```python
from build123d import *

# Parameters (mm, degrees)
F0_W      = 173
F0_H      = 50
F1_DEPTH  = 1.5
F2_W      = 1.5
F2_H      = 4.5
F4_DEPTH  = 1.501
F3_W      = 1.5
F3_H      = 4.5
F5_DEPTH  = 1.501
F6_W      = 4
F6_H      = 2.7
F7_DEPTH  = 1.501
F8_R      = 1.35
F9_DEPTH  = 1.501
F10_R     = 3.75
F11_DEPTH = 1.501
F12_W     = 4
F12_H     = 1.2
F13_DEPTH = 1.501
F14_W     = 1.4
F14_H     = 4
F15_DEPTH = 1.501
F16_R     = 1
F17_R     = 0.5
F18_DEPTH = 1.501
F19_W     = 1.5543582849
F19_H     = 10.2004739456
F20_DEPTH = 1.501


# Not quite as in the source:
# - a pattern or mirror of a feature is missing from the dataset's text; its kind, count and spacing are read off the source's solid


with BuildPart() as f1:
    # F0 (on Top) → F1 (new body)
    with BuildSketch(Plane.XY):
        Rectangle(F0_W, F0_H)
    extrude(amount=F1_DEPTH)

    # F2 (on face) → F4 (cut, through all)
    with BuildSketch(Plane.XY.offset(1.5)):
        with Locations((-69.95, 2.75)):
            Rectangle(F2_W, F2_H)
    extrude(amount=-F4_DEPTH, mode=Mode.SUBTRACT)

    # F3 (on face) → F5 (cut, through all)
    with BuildSketch(Plane.XY.offset(1.5)):
        with Locations((-55.25, 2.75)):
            Rectangle(F3_W, F3_H)
    extrude(amount=-F5_DEPTH, mode=Mode.SUBTRACT)

    # F6 (on face) → F7 (cut, through all)
    with BuildSketch(Plane.XY.offset(1.5)):
        with Locations((-18.5, 20.65)):
            Rectangle(F6_W, F6_H)
    f7 = extrude(amount=-F7_DEPTH, mode=Mode.SUBTRACT)

    # F7_copies: F7 across plane
    add(f7.mirror(Plane(origin=(0, 0, 0), x_dir=(0, 0, -1), z_dir=(0, -1, 0))), mode=Mode.SUBTRACT)

    # F8 (on face) → F9 (cut, through all)
    with BuildSketch(Plane.XY.offset(1.5)):
        with Locations((56.55, 20.45)):
            Circle(F8_R)
    f9 = extrude(amount=-F9_DEPTH, mode=Mode.SUBTRACT)

    # F9_copies: F9 across plane
    add(f9.mirror(Plane(origin=(0, 0, 0), x_dir=(0, 0, -1), z_dir=(0, -1, 0))), mode=Mode.SUBTRACT)

    # F10 (on face) → F11 (cut, through all)
    with BuildSketch(Plane.XY.offset(1.5)):
        with Locations((76.35, 16.45)):
            Circle(F10_R)
        with Locations((76.35, -11.75)):
            Circle(F10_R)
    extrude(amount=-F11_DEPTH, mode=Mode.SUBTRACT)

    # F12 (on face) → F13 (cut, through all)
    with BuildSketch(Plane.XY.offset(1.5)):
        with Locations((84.5, 8.2552298188)):
            Rectangle(F12_W, F12_H)
        with Locations((84.5, -2.9447701812)):
            Rectangle(F12_W, F12_H)
    extrude(amount=-F13_DEPTH, mode=Mode.SUBTRACT)

    # F14 (on face) → F15 (cut, through all)
    with BuildSketch(Plane.XY.offset(1.5)):
        with Locations((75.6, 2.8)):
            Rectangle(F14_W, F14_H)
    extrude(amount=-F15_DEPTH, mode=Mode.SUBTRACT)

    # F16
    f16_edges = [f1.edges().sort_by_distance(p)[0] for p in [
        (-86.5, -25, 0.75),
        (-86.5, 25, 0.75),
        (86.5, 25, 0.75),
        (86.5, -25, 0.75),
    ]]
    fillet(f16_edges, radius=F16_R)

    # F17 (on face) → F18 (cut, through all)
    with BuildSketch(Plane.XY.offset(1.5)):
        with Locations((-25.3, -2.5)):
            Circle(F17_R)
        with Locations((-22.9, -2.5)):
            Circle(F17_R)
        with Locations((-20.5, -2.5)):
            Circle(F17_R)
        with Locations((-20.5, -8.5)):
            Circle(F17_R)
        with Locations((-22.9, -8.5)):
            Circle(F17_R)
        with Locations((-25.3, -8.5)):
            Circle(F17_R)
    extrude(amount=-F18_DEPTH, mode=Mode.SUBTRACT)

    # F19 (on face) → F20 (cut, through all)
    with BuildSketch(Plane.XY.offset(1.5)):
        with Locations((-7.3602499906, -0.7336952258)):
            Rectangle(F19_W, F19_H)
    extrude(amount=-F20_DEPTH, mode=Mode.SUBTRACT)


solid = f1.part
```
CAD build for the part. Positions are in the model's coordinates, mm. Round coordinates to 2 decimals unless told otherwise and drop trailing zeros. Loops run counter-clockwise (first coordinate to the right, second up) from the corner with the lowest first, then second, coordinate; pieces in that order, holes last. Notation, with made-up numbers: M 61,-26 L 80,-26 A26 ccw 80,-5 Z; hole C 48,-28 d10. An arc over 180 degrees is marked long. Use a Markdown table: item, result. Add a question column.
(1) Cut at A-A (y = -14). Give the cut face in (x, z), and give its area (4 significant figures).
(2) Drill centre lines: line 1 (X direction, y = -20.45, z = 1.15); line 2 (Y direction, x = -22.9, z = 0.4); line 3 (X direction, y = 19.5, z = 1.3). Where is each one in solid material? Low to high.
(3) Cut at B-B (z = 0.35). State how many separate pieces and enclosed holes the cut face has, and give its area (3 significant figures).
(4) Flat gauge pin, fed straight in: pin 1 (0.6 mm diameter, centred on y = -3, z = 1, fed in from +X). Where does the tip first touch, or does it go through?
(5) Pull direction X, two halves, no side cores. Call faces 1 (the face through (79.927, -10.624, 0.76)), 2 (the face through (-1, 0, 1.5)), 3 (the face through (79.814, 15.014, 0.76)): +X half, -X half, draft (parallel to the pull), parting line (faces both ways), or undercut.
Geometry says:
| question | item | result |
|---|---|---|
| 1 | outline | M -86.5,0 L 73.35,0 L 73.35,1.5 L -86.5,1.5 Z; M 79.35,0 L 86.5,0 L 86.5,1.5 L 79.35,1.5 Z |
| 1 | area | 250.5 mm² |
| 2 | line 1 | x = -86.5 to -20.5, -16.5 to 55.2, 57.9 to 86.5 |
| 2 | line 2 | y = -25 to -9, -8 to -3, -2 to 25 |
| 2 | line 3 | x = -86.5 to -20.5, -16.5 to 55.59, 57.51 to 74.17, 78.53 to 86.5 |
| 3 | separate pieces | 1 |
| 3 | enclosed holes | 16 |
| 3 | area | 8,480 mm² |
| 4 | pin 1 | stops at x = 82.5 |
| 5 | face 1 | undercut |
| 5 | face 2 | draft |
| 5 | face 3 | undercut |
